```python
from build123d import *

# Parameters (mm, degrees)
CROQUIS1_R              = 1.75
SALIENTE_EXTRUIR1_DEPTH = 3


with BuildPart() as part:
    # Croquis1 → Saliente-Extruir1 (new body)
    with BuildSketch(Plane(origin=(0, 0, 0), x_dir=(0, 0, -1), z_dir=(1, 0, 0))):
        with BuildLine():
            Line((-23.535533906, 23.535533906), (-15.90493831, 31.166129502))
            Line((-15.90493831, 31.166129502), (-13.783617966, 29.044809158))
            Line((-13.783617966, 29.044809158), (-6.712550154, 36.11587697))
            Line((-6.712550154, 36.11587697), (-8.833870498, 38.237197314))
            Line((-8.833870498, 38.237197314), (-0.121320344, 46.949747468))
            ThreePointArc((-0.121320344, 46.949747468), (3.148050297, 47.600065722), (5, 44.828427125))
            Line((5, 44.828427125), (5, 0))
            ThreePointArc((5, 0), (-1.125347327, -4.871713599), (-4.493437357, 2.192947952))
            ThreePointArc((-4.493437357, 2.192947952), (-9.426479438, 10.796864219), (-18.255804358, 15.314086902))
            ThreePointArc((-18.255804358, 15.314086902), (-24.207168989, 17.298198916), (-23.535533906, 23.535533906))
        make_face()
        Circle(CROQUIS1_R, mode=Mode.SUBTRACT)
        with Locations((-20, 20)):
            Circle(CROQUIS1_R, mode=Mode.SUBTRACT)
    extrude(amount=SALIENTE_EXTRUIR1_DEPTH)


solid = part.part
```
Input: part model. Units: mm. Frame: model coordinates. A direction names the side the tool comes from. Give positions to 0.01 mm unless a question says otherwise; leave off trailing zeros. Order: outer loops, then holes, each group sorted by start corner. A loop starts at its lowest first (then second) coordinate and runs counter-clockwise, first axis right, second up. Notation, with made-up numbers: (58.5, -32.5) - (79.5, -32.5) arc R10 ccw to (79.5, -27.5) - close; hole circle Ø4 at (61, 29.25). An arc over 180 degrees is marked (long way). One line per item, written item: value.
1. Draft query along Z for faces 6 (the face through (1.48, 47.62, -3.1)), 7 (the face through (1, 23, -5)), 8 (the face through (1.479, -0.67, -1.617)). Return one class per face: released by +Z, released by -Z, zero draft, split by the parting line, or undercut.
Determined:
face 6: split by the parting line
face 7: released by -Z
face 8: undercut
2. Line query: probe 1 along Z at (x, y) = (1, 21.5); probe 2 along Y at (x, z) = (0.15, 8.5); probe 3 along Y at (x, z) = (0.7, 20). Output: solid intervals per line, ascending.
Determined:
probe 1: -5 to 19.1, 20.9 to 24.77
probe 2: 9.84 to 34.33, 37.9 to 38.57
probe 3: 15 to 18.25, 21.75 to 27.07
3. Cut plane A-A, the plane x = 1.2. Output: boundary loops of the cut face in (y, z), and give its area (3 significant figures).
Determined:
outline: (0, -5) - (44.83, -5) arc R3 ccw to (46.95, 0.12) - (38.24, 8.83) - (36.12, 6.71) - (29.04, 13.78) - (31.17, 15.9) - (23.54, 23.54) arc R5 ccw to (15.31, 18.26) arc R17.42 cw to (2.19, 4.49) arc R5 ccw (long way) to start; hole circle Ø3.5 at (0, 0); hole circle Ø3.5 at (20, 20)
area: 828 mm2
4. Reachability of faces 1 (the face through (1.48, 30.12, 14.86)), 2 (the face through (1.48, 27.3, 19.77)), 3 (the face through (1.479, 37.162, 7.758)), 4 (the face through (1.48, 32.53, 10.3)), 5 (the face through (3, 22, 6)) from +Z, -Z, +X, -X, +Y, -Y: full face, straight path, thin tool, end or side. Return the list, or none.
Determined:
face 1: +X, -X, +Y
face 2: +Z, +X, -X, +Y
face 3: +Z, +X, -X
face 4: +X, -X
face 5: +Z, -Z, +X, +Y, -Y
5. Cut plane D-D, the plane y = 10. Output: boundary loops of the cut face in (x, z).
Determined:
outline: (0, -5) - (3, -5) - (3, 8.64) - (0, 8.64) - close
6. Cut plane C-C, the plane z = 8. Output: boundary loops of the cut face in (x, y), and give its area (3 significant figures).
Determined:
outline: (0, 9.26) - (3, 9.26) - (3, 34.83) - (0, 34.83) - close; (0, 37.4) - (3, 37.4) - (3, 39.07) - (0, 39.07) - close
area: 81.7 mm2
7. Cut plane B-B, the plane y = 20. Output: boundary loops of the cut face in (x, z), and give its area (3 significant figures).
Determined:
outline: (0, -5) - (3, -5) - (3, 18.25) - (0, 18.25) - close; (0, 21.75) - (3, 21.75) - (3, 25) - (0, 25) - close
area: 79.5 mm2
